For this review, take the finished solid that the model builds, in its own axes (mm). Give positions to 0.01 mm unless a question says otherwise; leave off trailing zeros. Order: outer loops, then holes, each group sorted by start corner. A loop starts at its lowest first (then second) coordinate and runs counter-clockwise, first axis right, second up. Notation, with made-up numbers: (-7.75, -37) -> (44.25, -37) arc R32 cw to (44.25, -3) -> close; hole circle Ø4 at (32, -11.75). An arc over 180 degrees is marked (long way). Return JSON: item names as keys, results as strings. Group by question number.
1) The part is to be moulded in two halves that separate along Y. For faces 1 (the face through (0, -8.89, -1)), 2 (the face through (-15.24, 0, -1)), 3 (the face through (13.56, 7.89, -0.81)), 4 (the face through (-13.97, 0.06, -0.81)), say which applies: released by +Y, released by -Y, zero draft, split by the parting line, or undercut.
2) Add section B-B (x = -12.7). Give the boundary of the cut face in (y, z), then the cut area to 3 significant figures.
3) Add section A-A (y = 0). Give the boundary of the cut face in (x, z), then the cut area to 3 significant figures.
4) To check wall thickness, follow line 1 along Y through (x, z) = (0, -1.3); line 2 along Y through (x, z) = (-2.5, -0.6); line 3 along Y through (x, z) = (13, -1.5). State the ranges of each line that lie inside material, in increasing order.
5) Add section C-C (x = 0). Give the boundary of the cut face in (y, z).
6) Add section D-D (z = -0.95). State how many separate pieces and enclosed holes the cut face has, then the cut area to 3 significant figures.
from build123d import *

# Parameters (mm, degrees)
SKETCH040_W            = 30.48
SKETCH040_H            = 17.78
PAD015_DEPTH           = 1.65
SKETCH042_R            = 1.27
POCKET024_DEPTH        = 1.651
SKETCH044_R            = 0.4
POCKET025_DEPTH        = 1.651
LINEARPATTERN_COUNT    = 12
LINEARPATTERN_PITCH    = 2.770909
LINEARPATTERN001_COUNT = 12
LINEARPATTERN001_PITCH = 2.770909


with BuildPart() as part:
    # Sketch040 → Pad015 (new body)
    with BuildSketch(Plane.XY):
        Rectangle(SKETCH040_W, SKETCH040_H)
    extrude(amount=-PAD015_DEPTH)

    # Sketch042 → Pocket024 (cut, through all)
    with BuildSketch(Plane.XY):
        with Locations((-12.7, 0)):
            Circle(SKETCH042_R)
        with Locations((12.7, 0)):
            Circle(SKETCH042_R)
    extrude(amount=-POCKET024_DEPTH, mode=Mode.SUBTRACT)

    # Sketch044 → Pocket025 (cut, through all)
    with BuildSketch(Plane.XY):
        with Locations((0, -7.62)):
            Circle(SKETCH044_R)
        with Locations((0, 7.62)):
            Circle(SKETCH044_R)
    pocket025 = extrude(amount=-POCKET025_DEPTH, mode=Mode.SUBTRACT)

    # LinearPattern: Pocket025 ×12
    with Locations(*[(i * LINEARPATTERN_PITCH, 0, 0) for i in range(1, LINEARPATTERN_COUNT)]):
        add(pocket025, mode=Mode.SUBTRACT)

    # LinearPattern001: Pocket025 ×12
    with Locations(*[(-i * LINEARPATTERN001_PITCH, 0, 0) for i in range(1, LINEARPATTERN001_COUNT)]):
        add(pocket025, mode=Mode.SUBTRACT)


solid = part.part
Evaluation:
{
 "1": {"face 1": "released by -Y", "face 2": "zero draft", "face 3": "undercut", "face 4": "undercut"},
 "2": {"outline": "(-8.89, -1.65) -> (-1.27, -1.65) -> (-1.27, 0) -> (-8.89, 0) -> close; (1.27, -1.65) -> (8.89, -1.65) -> (8.89, 0) -> (1.27, 0) -> close", "area": "25.1 mm^2"},
 "3": {"outline": "(-15.24, -1.65) -> (-13.97, -1.65) -> (-13.97, 0) -> (-15.24, 0) -> close; (-11.43, -1.65) -> (11.43, -1.65) -> (11.43, 0) -> (-11.43, 0) -> close; (13.97, -1.65) -> (15.24, -1.65) -> (15.24, 0) -> (13.97, 0) -> close", "area": "41.9 mm^2"},
 "4": {"line 1": "-8.89 to -8.02, -7.22 to 7.22, 8.02 to 8.89", "line 2": "-8.89 to -7.91, -7.33 to 7.33, 7.91 to 8.89", "line 3": "-8.89 to -1.23, 1.23 to 8.89"},
 "5": {"outline": "(-8.89, -1.65) -> (-8.02, -1.65) -> (-8.02, 0) -> (-8.89, 0) -> close; (-7.22, -1.65) -> (7.22, -1.65) -> (7.22, 0) -> (-7.22, 0) -> close; (8.02, -1.65) -> (8.89, -1.65) -> (8.89, 0) -> (8.02, 0) -> close"},
 "6": {"separate pieces": "1", "enclosed holes": "24", "area": "521 mm^2"}
}
